from build123d import *

# Parameters (mm, degrees)
F0_W     = 10.6189064682
F0_H     = 22.5
F0_W_2   = 25.791388005
F0_H_2   = 3.9892950654
F1_DEPTH = 30


with BuildPart() as f1:
    # F0 (on Front) → F1 (new body, symmetric)
    with BuildSketch(Plane.XZ):
        Polygon((-61.6173371673, 30), (-61.6173371673, 22.5), (-20.9044199437, 15), (-20.9044199437, 0), (-20.9044199437, -15), (-61.6173371673, -22.5), (-61.6173371673, -30), (0, -30), (36.4102944732, -30), (36.4102944732, -26.4892950654), (25.791388005, -26.4892950654), (25.791388005, -22.5), (0, -22.5), (0, 0), (0, 22.5), (25.791388005, 22.5), (25.791388005, 26.4892950654), (36.4102944732, 26.4892950654), (36.4102944732, 30), (0, 30), align=None)
        with Locations((31.1008412391, 11.25)):
            Rectangle(F0_W, F0_H)
        with Locations((12.8956940025, 11.25)):
            Rectangle(F0_W_2, F0_H)
        Polygon((-20.9044199437, 15), (-61.6173371673, 22.5), (-61.6173371673, 0), (-20.9044199437, 0), align=None)
        Polygon((-20.9044199437, 0), (-61.6173371673, 0), (-61.6173371673, -22.5), (-20.9044199437, -15), align=None)
        with Locations((31.1008412391, -11.25)):
            Rectangle(F0_W, F0_H)
        with Locations((12.8956940025, -11.25)):
            Rectangle(F0_W_2, F0_H)
        with Locations((31.1008412391, 24.4946475327)):
            Rectangle(F0_W, F0_H_2)
        with Locations((31.1008412391, -24.4946475327)):
            Rectangle(F0_W, F0_H_2)
    extrude(amount=F1_DEPTH, both=True)

    # F0 (on Front) → F2 (revolve, cut)
    with BuildSketch(Plane.XZ):
        Polygon((-20.9044199437, 0), (-61.6173371673, 0), (-61.6173371673, -22.5), (-20.9044199437, -15), align=None)
    revolve(axis=Axis((-6.6388677806, 0, 0), (1, 0, 0)), mode=Mode.SUBTRACT)

    # F0 (on Front) → F3 (revolve, cut)
    with BuildSketch(Plane.XZ):
        with Locations((31.1008412391, 11.25)):
            Rectangle(F0_W, F0_H)
        with Locations((12.8956940025, 11.25)):
            Rectangle(F0_W_2, F0_H)
        with Locations((31.1008412391, 24.4946475327)):
            Rectangle(F0_W, F0_H_2)
    revolve(axis=Axis((-6.6388677806, 0, 0), (1, 0, 0)), mode=Mode.SUBTRACT)


solid = f1.part
The model under review builds one solid part; all positions refer to its coordinate system, in mm. A direction names the side the tool comes from. Give positions to 0.01 mm unless a question says otherwise; leave off trailing zeros. Order: outer loops, then holes, each group sorted by start corner. A loop starts at its lowest first (then second) coordinate and runs counter-clockwise, first axis right, second up. Notation, with made-up numbers: M -33,-35 L 13,-35 A13 cw 13,-30 Z; hole C -34.5,52.5 d10. An arc over 180 degrees is marked long. Use one line per item in the form item = value. Start each with the question number.
Item 1: Insertion check: pin 1 Ø3 at (y, z) = (9.5, -7) entering from -X; pin 2 Ø13.5 at (y, z) = (5.5, -9) entering from +X. Each pin has a flat end and moves straight along its axis. Give the tip position at first contact, or say it passes through.
Item 2: The part is to be moulded in two halves that separate along Z. For faces 4 (the flat face through (25.791, 19.5, 11.9)), 5 (the flat face through (-13, 30, 0)), 6 (the flat face through (-13, 0, -30)), say which applies: pulls with the +Z half, pulls with the -Z half, needs draft (parallel to the pull), parting line crosses it, or undercut.
Item 3: To check wall thickness, follow line 1 along Y through (x, z) = (30, 0); line 2 along Y through (x, z) = (16.5, 0). State the ranges of each line that lie inside material, in increasing order. Write a range as from..to.
Item 4: We need section D-D on x = 28.5. Give the boundary of the cut face in (y, z), plus the area to 3 significant figures.
Item 5: For faces 1 (the cylindrical face through (12.715, 19.961, 10.382)), 2 (the flat face through (-20.904, 0, 0)), 3 (the flat face through (-61.617, -20, 14)), list the 3-axis set-ups (+Z, -Z, +X, -X, +Y, -Y) from which the entire face can be reached by the end or side of a thin tool; tool diameter is ignored.
Item 6: We need section A-A on x = 5. Give the boundary of the cut face in (y, z).
Item 7: We need section B-B on z = 0. Give the boundary of the cut face in (x, y), plus the area to 3 significant figures.
Completed:
q1.pin_1 = -20.9
q1.pin_2 = 0
q2.face_4 = undercut
q2.face_5 = needs draft
q2.face_6 = pulls with the -Z half
q3.line_1 = -30..-26.49, 26.49..30
q3.line_2 = -30..-22.5, 22.5..30
q4.outline = M -30,-30 L 30,-30 L 30,30 L -30,30 Z; hole C 0,0 d52.98
q4.area = 1,400 mm²
q5.face_1 = +X
q5.face_2 = -X
q5.face_3 = +Z, -Z, -X, +Y, -Y
q6.outline = M -30,-30 L 30,-30 L 30,30 L -30,30 Z; hole C 0,0 d45
q7.outline = M -61.62,-30 L 36.41,-30 L 36.41,-26.49 L 25.79,-26.49 L 25.79,-22.5 L 0,-22.5 L 0,22.5 L 25.79,22.5 L 25.79,26.49 L 36.41,26.49 L 36.41,30 L -61.62,30 L -61.62,22.5 L -20.9,15 L -20.9,-15 L -61.62,-22.5 Z
q7.area = 2,630 mm²
